Build history of the part. All positions in model axes, mm. Coordinates: 2 decimals unless noted, no trailing zeros.
(1) Two-plate mould, pull along X, no slides. Class faces 1 (the face through (-30.456, 22.565, -1.642)), 2 (the face through (29.98, 22.56, 5.6)), 3 (the face through (-18.577, 22.565, -22.693)): pulls with the +X half, pulls with the -X half, needs draft (parallel to the pull), parting line crosses it, or undercut.
(2) Wall check: L1, parallel to X at y = 9.5, z = 23.5; L2, parallel to X at y = 39.5, z = -22; L3, parallel to Z at x = 21, y = 30.5. Give the ranges that are in metal, low to high.
(3) Flat gauge pins, fed straight in: P1, Ø1.5, axis at y = 15, z = 10, coming from the +X side; P2, Ø10, axis at y = 17.5, z = -22.5, coming from the -X side; P3, Ø5, axis at y = 9, z = 18.5, coming from the -X side. Where does each tip first touch, or does it go through?
from build123d import *

# Parameters (mm, degrees)
SKETCH1_R           = 27.131966011
BOSS_EXTRUDE1_DEPTH = 45.77


with BuildPart() as part:
    # Sketch1 → Boss-Extrude1 (new body)
    with BuildSketch(Plane(origin=(0, 0, 0), x_dir=(1, 0, 0), z_dir=(0, 1, 0))):
        with BuildLine():
            Line((-3.984261156, 27.848398027), (-3.155526874, 30.336328812))
            ThreePointArc((-3.155526874, 30.336328812), (-2.335703763, 30.410437264), (-1.5141793, 30.462394497))
            Line((-1.5141793, 30.462394497), (-0.315230151, 28.130201914))
            Line((-0.315230151, 28.130201914), (0.831154566, 30.48867707))
            ThreePointArc((0.831154566, 30.48867707), (1.65363686, 30.455143124), (2.474914637, 30.399425407))
            Line((2.474914637, 30.399425407), (3.359194573, 27.930690283))
            Line((3.359194573, 27.930690283), (4.803614875, 30.119355554))
            ThreePointArc((4.803614875, 30.119355554), (9.479661295, 28.989418191), (13.919878882, 27.138300594))
            Line((13.919878882, 27.138300594), (13.792102919, 24.51908612))
            Line((13.792102919, 24.51908612), (15.964140245, 25.988394149))
            ThreePointArc((15.964140245, 25.988394149), (16.659663243, 25.548112068), (17.343051232, 25.089220567))
            Line((17.343051232, 25.089220567), (16.874492259, 22.509091617))
            Line((16.874492259, 22.509091617), (19.21973095, 23.682321883))
            ThreePointArc((19.21973095, 23.682321883), (19.851835217, 23.155022565), (20.469479277, 22.610856977))
            Line((20.469479277, 22.610856977), (19.668154402, 20.113960352))
            Line((19.668154402, 20.113960352), (22.146466743, 20.971038467))
            ThreePointArc((22.146466743, 20.971038467), (22.704336831, 20.365744156), (23.245668935, 19.745615304))
            Line((23.245668935, 19.745615304), (22.125289014, 17.374673686))
            Line((22.125289014, 17.374673686), (24.69427034, 17.900934736))
            ThreePointArc((24.69427034, 17.900934736), (25.168360968, 17.228002177), (25.624118803, 16.542520632))
            Line((25.624118803, 16.542520632), (24.203853841, 14.338101571))
            Line((24.203853841, 14.338101571), (26.8195481, 14.52454104))
            ThreePointArc((26.8195481, 14.52454104), (27.201747469, 13.795484281), (27.564132913, 13.056378805))
            Line((27.564132913, 13.056378805), (25.868284062, 11.0562006))
            Line((25.868284062, 11.0562006), (28.485935925, 10.899628442))
            ThreePointArc((28.485935925, 10.899628442), (28.769704511, 10.126921824), (29.032517063, 9.346838694))
            Line((29.032517063, 9.346838694), (27.090100815, 7.585125008))
            Line((27.090100815, 7.585125008), (29.664921456, 7.088220232))
            ThreePointArc((29.664921456, 7.088220232), (29.845403904, 6.285084953), (30.00414677, 5.47737158))
            Line((30.00414677, 5.47737158), (27.848398476, 3.984265861))
            Line((27.848398476, 3.984265861), (30.336331931, 3.15553069))
            ThreePointArc((30.336331931, 3.15553069), (30.410440131, 2.33570859), (30.462397167, 1.514185147))
            Line((30.462397167, 1.514185147), (28.130202362, 0.315234856))
            Line((28.130202362, 0.315234856), (30.488679348, -0.83115075))
            ThreePointArc((30.488679348, -0.83115075), (30.455145268, -1.653632314), (30.399427457, -2.474909359))
            Line((30.399427457, -2.474909359), (27.930690731, -3.359189868))
            Line((27.930690731, -3.359189868), (30.11935702, -4.803610841))
            ThreePointArc((30.11935702, -4.803610841), (29.97875441, -5.614679004), (29.81631507, -6.421657392))
            Line((29.81631507, -6.421657392), (27.253277282, -6.976137886))
            Line((27.253277282, -6.976137886), (29.234684181, -8.693879674))
            ThreePointArc((29.234684181, -8.693879674), (28.989418755, -9.479656851), (28.723037229, -10.258528973))
            Line((28.723037229, -10.258528973), (26.109552746, -10.473722214))
            Line((26.109552746, -10.473722214), (27.849797859, -12.435393664))
            ThreePointArc((27.849797859, -12.435393664), (27.504066132, -13.182434995), (27.138300238, -13.919874138))
            Line((27.138300238, -13.919874138), (24.519086569, -13.792098214))
            Line((24.519086569, -13.792098214), (25.988393872, -15.964134468))
            ThreePointArc((25.988393872, -15.964134468), (25.548111361, -16.659657866), (25.089219408, -17.343046235))
            Line((25.089219408, -17.343046235), (22.509092066, -16.874487554))
            Line((22.509092066, -16.874487554), (23.682321388, -19.219724361))
            ThreePointArc((23.682321388, -19.219724361), (20.365742572, -22.704330231), (16.542517807, -25.624111989))
            Line((16.542517807, -25.624111989), (14.33810202, -24.203849136))
            Line((14.33810202, -24.203849136), (14.524541185, -26.819539129))
            ThreePointArc((14.524541185, -26.819539129), (13.795482869, -27.201739208), (13.056375797, -27.564125279))
            Line((13.056375797, -27.564125279), (11.056201049, -25.868279357))
            Line((11.056201049, -25.868279357), (10.899629182, -28.485926359))
            ThreePointArc((10.899629182, -28.485926359), (10.126920725, -28.76969554), (9.346835723, -29.032508588))
            Line((9.346835723, -29.032508588), (7.585125457, -27.09009611))
            Line((7.585125457, -27.09009611), (7.0882217, -29.66491147))
            ThreePointArc((7.0882217, -29.66491147), (6.285084339, -29.845394329), (5.477368862, -30.004137493))
            Line((5.477368862, -30.004137493), (3.984266309, -27.848393771))
            Line((3.984266309, -27.848393771), (3.15553297, -30.336321728))
            ThreePointArc((3.15553297, -30.336321728), (2.3357086, -30.410430097), (1.51418288, -30.462387181))
            Line((1.51418288, -30.462387181), (0.315235305, -28.130197658))
            Line((0.315235305, -28.130197658), (-0.831147629, -30.488669145))
            ThreePointArc((-0.831147629, -30.488669145), (-1.653631581, -30.455134954), (-2.474911005, -30.399416902))
            Line((-2.474911005, -30.399416902), (-3.35918942, -27.930686027))
            Line((-3.35918942, -27.930686027), (-4.803606908, -30.119347035))
            ThreePointArc((-4.803606908, -30.119347035), (-5.614677501, -29.978744012), (-6.421658293, -29.816304126))
            Line((-6.421658293, -29.816304126), (-6.976137437, -27.253272577))
            Line((-6.976137437, -27.253272577), (-8.693875013, -29.234674617))
            ThreePointArc((-8.693875013, -29.234674617), (-9.479654581, -28.989408474), (-10.258529053, -28.723026103))
            Line((-10.258529053, -28.723026103), (-10.473721765, -26.109548042))
            Line((-10.473721765, -26.109548042), (-12.435388408, -27.84978889))
            ThreePointArc((-12.435388408, -27.84978889), (-13.182432016, -27.504056163), (-13.919873378, -27.138289149))
            Line((-13.919873378, -27.138289149), (-13.792097766, -24.519081864))
            Line((-13.792097766, -24.519081864), (-15.964128792, -25.988385631))
            ThreePointArc((-15.964128792, -25.988385631), (-16.659654283, -25.548101878), (-17.343044673, -25.089208572))
            Line((-17.343044673, -25.089208572), (-16.874487106, -22.509087361))
            Line((-16.874487106, -22.509087361), (-19.219718467, -23.68231396))
            ThreePointArc((-19.219718467, -23.68231396), (-19.851825173, -23.155012543), (-20.469471557, -22.610844724))
            Line((-20.469471557, -22.610844724), (-19.668149248, -20.113956096))
            Line((-19.668149248, -20.113956096), (-22.146453419, -20.971031386))
            ThreePointArc((-22.146453419, -20.971031386), (-22.704325784, -20.365734574), (-23.245660027, -19.745603103))
            Line((-23.245660027, -19.745603103), (-22.125283861, -17.374669429))
            Line((-22.125283861, -17.374669429), (-24.694256422, -17.900928684))
            ThreePointArc((-24.694256422, -17.900928684), (-25.168349066, -17.227993282), (-25.62410876, -16.542508787))
            Line((-25.62410876, -16.542508787), (-24.203848687, -14.338097315))
            Line((-24.203848687, -14.338097315), (-26.819533875, -14.524536138))
            ThreePointArc((-26.819533875, -14.524536138), (-27.201734918, -13.79547627), (-27.564121868, -13.056367599))
            Line((-27.564121868, -13.056367599), (-25.868278909, -11.056196344))
            Line((-25.868278909, -11.056196344), (-28.4859217, -10.899624729))
            ThreePointArc((-28.4859217, -10.899624729), (-29.845390828, -6.285079097), (-30.462384511, -1.514177033))
            Line((-30.462384511, -1.514177033), (-28.130197209, -0.3152306))
            Line((-28.130197209, -0.3152306), (-30.488666867, 0.831151445))
            ThreePointArc((-30.488666867, 0.831151445), (-30.455132809, 1.653636127), (-30.399414852, 2.474916284))
            Line((-30.399414852, 2.474916284), (-27.930685578, 3.359194124))
            Line((-27.930685578, 3.359194124), (-30.119345569, 4.803610941))
            ThreePointArc((-30.119345569, 4.803610941), (-29.978742638, 5.614681962), (-29.816302822, 6.421663183))
            Line((-29.816302822, 6.421663183), (-27.253272129, 6.976142142))
            Line((-27.253272129, 6.976142142), (-29.23467388, 8.693879467))
            ThreePointArc((-29.23467388, 8.693879467), (-28.989407866, 9.479659161), (-28.72302562, 10.258533761))
            Line((-28.72302562, 10.258533761), (-26.109547593, 10.47372647))
            Line((-26.109547593, 10.47372647), (-27.849788746, 12.435393457))
            ThreePointArc((-27.849788746, 12.435393457), (-27.504056265, 13.182436908), (-27.138289505, 13.919878122))
            Line((-27.138289505, 13.919878122), (-24.519081415, 13.792102471))
            Line((-24.519081415, 13.792102471), (-25.988385908, 15.964134569))
            ThreePointArc((-25.988385908, 15.964134569), (-25.548102584, 16.65965966), (-25.089209731, 17.34304967))
            Line((-25.089209731, 17.34304967), (-22.509086912, 16.87449181))
            Line((-22.509086912, 16.87449181), (-23.682314454, 19.219725057))
            ThreePointArc((-23.682314454, 19.219725057), (-23.155013707, 19.851831175), (-22.610846592, 20.469477005))
            Line((-22.610846592, 20.469477005), (-20.113955647, 19.668153953))
            Line((-20.113955647, 19.668153953), (-20.97103188, 22.14646085))
            ThreePointArc((-20.97103188, 22.14646085), (-20.36573602, 22.704332508), (-19.745605539, 23.245666095))
            Line((-19.745605539, 23.245666095), (-17.374668981, 22.125288565))
            Line((-17.374668981, 22.125288565), (-17.90092896, 24.694264665))
            ThreePointArc((-17.90092896, 24.694264665), (-17.227994811, 25.168356561), (-16.542511612, 25.624115574))
            Line((-16.542511612, 25.624115574), (-14.338096867, 24.203853392))
            Line((-14.338096867, 24.203853392), (-14.524535993, 26.819542846))
            ThreePointArc((-14.524535993, 26.819542846), (-13.795477682, 27.20174318), (-13.056370606, 27.564129503))
            Line((-13.056370606, 27.564129503), (-11.056195896, 25.868283613))
            Line((-11.056195896, 25.868283613), (-10.89962399, 28.485931265))
            ThreePointArc((-10.89962399, 28.485931265), (-10.126915935, 28.769700534), (-9.346831335, 29.032513688))
            Line((-9.346831335, 29.032513688), (-7.585120303, 27.090100366))
            Line((-7.585120303, 27.090100366), (-7.088216199, 29.664917524))
            ThreePointArc((-7.088216199, 29.664917524), (-6.06936901, 29.890013635), (-5.043418528, 30.08012798))
            Line((-5.043418528, 30.08012798), (-3.984261156, 27.848398027))
        make_face()
        with Locations(Location((2.577e-06, 2.128e-06, 0), (0, 0, 270))):
            Circle(SKETCH1_R, mode=Mode.SUBTRACT)
    extrude(amount=BOSS_EXTRUDE1_DEPTH)


solid = part.part
Response values:
1. face 1: pulls with the -X half
1. face 2: pulls with the +X half
1. face 3: undercut
2. L1: x = -19.44 to -18.86, -17.05 to -13.56, 13.56 to 19.44
2. L2: x = -20.92 to -15.88, 15.88 to 20.27
2. L3: z = -20.57 to -17.18, 17.18 to 22.12
3. P1: stops at x = 29.06
3. P2: stops at x = -23.68
3. P3: stops at x = -25.62
